Design review of the part shown in the three views and the two pictorial views. Dimensions are in mm from the part's minimum x, y and z. A direction names the side the tool comes from. Give positions to 0.01 mm unless a question says otherwise; leave off trailing zeros. Loops run counter-clockwise (first coordinate to the right, second up) from the corner with the lowest first, then second, coordinate; pieces in that order, holes last.
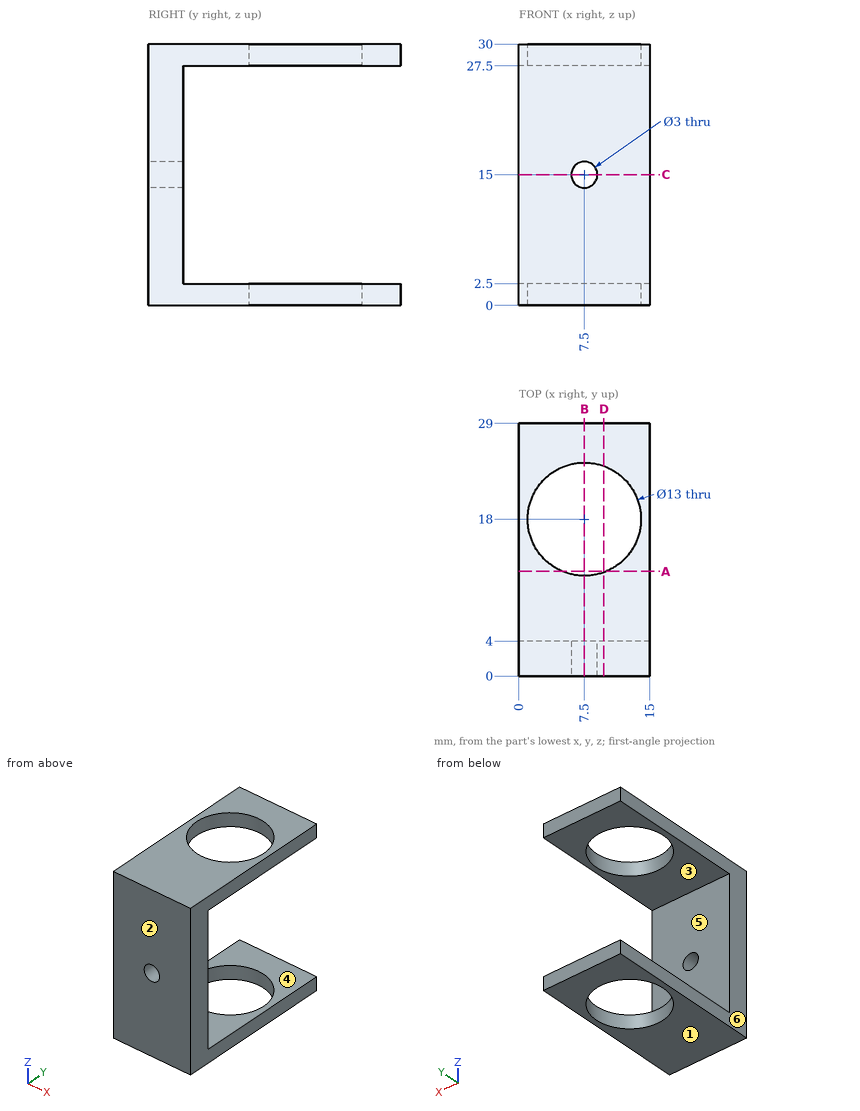
Q1. Consider section B-B on x = 7.5. Give the boundary of the cut face in (y, z), plus the area to 3 significant figures.
Answers:
outline: (0, 0) - (11.5, 0) - (11.5, 2.5) - (4, 2.5) - (4, 13.5) - (0, 13.5) - close; (0, 16.5) - (4, 16.5) - (4, 27.5) - (11.5, 27.5) - (11.5, 30) - (0, 30) - close; (24.5, 0) - (29, 0) - (29, 2.5) - (24.5, 2.5) - close; (24.5, 27.5) - (29, 27.5) - (29, 30) - (24.5, 30) - close
area: 168 mm2
Q2. Consider section D-D on x = 9.75. Give the boundary of the cut face in (y, z), plus the area to 3 significant figures.
Answers:
outline: (0, 0) - (11.9, 0) - (11.9, 2.5) - (4, 2.5) - (4, 27.5) - (11.9, 27.5) - (11.9, 30) - (0, 30) - close; (24.1, 0) - (29, 0) - (29, 2.5) - (24.1, 2.5) - close; (24.1, 27.5) - (29, 27.5) - (29, 30) - (24.1, 30) - close
area: 184 mm2
Q3. For pin 1 Ø2.5 at (x, z) = (7.5, 15) entering from +Y; pin 2 Ø4.5 at (x, z) = (6.5, 19) entering from +Y, all flat-tipped, find the tip position at first contact; note any pin that passes through.
Answers:
pin 1: passes through
pin 2: stops at y = 4
Q4. Consider section C-C on z = 15. Give the boundary of the cut face in (x, y).
Answers:
outline: (0, 0) - (6, 0) - (6, 4) - (0, 4) - close; (9, 0) - (15, 0) - (15, 4) - (9, 4) - close
Q5. Mouldability with a two-part tool opening along Z and no side actions: class the marked faces 1, 2, 3 and 4 as +Z half, -Z half, draft (parallel to the pull), parting line (faces both ways), or undercut.
Answers:
face 1: -Z half
face 2: draft
face 3: undercut
face 4: undercut
Q6. Machinability: for the marked faces 5 and 6, which of the approach directions +Z, -Z, +X, -X, +Y, -Y give a long, thin tool a straight path to every point of the face, cutting with its end or side? Answer none if there is none.
Answers:
face 5: +X, -X, +Y
face 6: +Z, -Z, -X, +Y, -Y
Q7. For probe 1 along Y at (x, z) = (7.5, 0.55); probe 2 along Z at (x, y) = (7.5, 1.75); probe 3 along Z at (x, y) = (10.25, 11), list the stretches that pass through material, from the lowest coordinate up.
Answers:
probe 1: y = 0 to 11.5, 24.5 to 29
probe 2: z = 0 to 13.5, 16.5 to 30
probe 3: z = 0 to 2.5, 27.5 to 30
Q8. Consider section A-A on y = 12. Give the boundary of the cut face in (x, z), plus the area to 3 significant figures.
Answers:
outline: (0, 0) - (5, 0) - (5, 2.5) - (0, 2.5) - close; (0, 27.5) - (5, 27.5) - (5, 30) - (0, 30) - close; (10, 0) - (15, 0) - (15, 2.5) - (10, 2.5) - close; (10, 27.5) - (15, 27.5) - (15, 30) - (10, 30) - close
area: 50.0 mm2
